Verification items for the finished model (mm, model axes). Give positions to 0.01 mm unless a question says otherwise; leave off trailing zeros. Order: outer loops, then holes, each group sorted by start corner. A loop starts at its lowest first (then second) coordinate and runs counter-clockwise, first axis right, second up. Notation, with made-up numbers: (75.25, 2.25) - (117.25, 2.25) arc R25 ccw to (117.25, 21.25) - close; hole circle Ø4 at (-5, 69.5). An arc over 180 degrees is marked (long way). Answer as a JSON object with one key per item and string values. Group by question number.
(1) Thickness scan on line 1 (Z direction, x = 28.5, y = 27); line 2 (Z direction, x = 5.5, y = -28.5); line 3 (X direction, y = 1, z = -116). Record the ranges inside material, lowest first.
(2) Section check A-A (z = 374.5). Record the boundary of the cut face in (x, y), then the cut area to 3 significant figures.
(3) Depth check by flat-ended pin: pin 1 Ø8 at (x, z) = (9.5, 32) entering from -Y; pin 2 Ø3 at (x, y) = (-28, -30.5) entering from -Z; pin 3 Ø5 at (y, z) = (-10.5, 190) entering from -X. Enter the tip coordinate at first touch or a pass-through.
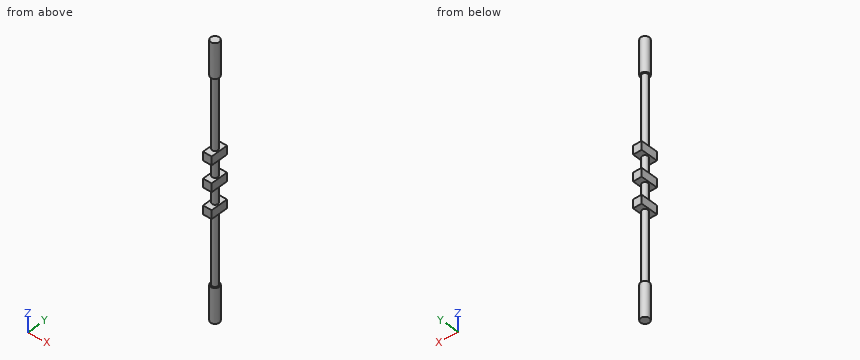
```python
from build123d import *

# Parameters (mm, degrees)
SKETCH1_R           = 25.4
BOSS_EXTRUDE1_DEPTH = 1778
SKETCH2_R           = 38.1
BOSS_EXTRUDE2_DEPTH = 304.8
BOSS_EXTRUDE3_START = 304.8
SKETCH3_R           = 38.1
BOSS_EXTRUDE3_DEPTH = 304.8
SKETCH4_W           = 76.2
SKETCH4_H           = 76.2
BOSS_EXTRUDE4_DEPTH = 76.2


with BuildPart() as part:
    # Sketch1 → Boss-Extrude1 (new body)
    with BuildSketch(Plane.XY):
        Circle(SKETCH1_R)
    extrude(amount=BOSS_EXTRUDE1_DEPTH)

    # Sketch2 → Boss-Extrude2 (add)
    with BuildSketch(Plane.XY.offset(1778)):
        with Locations(Location((0, 0, 0), (0, 0, 180))):
            Circle(SKETCH2_R)
    extrude(amount=BOSS_EXTRUDE2_DEPTH)

    # Sketch3 → Boss-Extrude3 (add)
    with BuildSketch(Plane(origin=(0, 0, 0), x_dir=(-1, 0, 0), z_dir=(0, 0, -1)).offset(BOSS_EXTRUDE3_START)):
        Circle(SKETCH3_R)
    extrude(amount=-BOSS_EXTRUDE3_DEPTH)

    # Sketch4 → Boss-Extrude4 (add, symmetric)
    with BuildSketch(Plane(origin=(0, 0, 0), x_dir=(1, 0, 0), z_dir=(0, 1, 0))):
        with Locations((0, -889)):
            Rectangle(SKETCH4_W, SKETCH4_H)
        with Locations((0, -1117.6)):
            Rectangle(SKETCH4_W, SKETCH4_H)
        with Locations((0, -660.4)):
            Rectangle(SKETCH4_W, SKETCH4_H)
    extrude(amount=BOSS_EXTRUDE4_DEPTH, both=True)


solid = part.part
```
Solutions:
{
 "1": {"line 1": "z = 622.3 to 698.5, 850.9 to 927.1, 1079.5 to 1155.7", "line 2": "z = -304.8 to 0, 622.3 to 698.5, 850.9 to 927.1, 1079.5 to 1155.7, 1778 to 2082.8", "line 3": "x = -38.09 to 38.09"},
 "2": {"outline": "circle Ø50.8 at (0, 0)", "area": "2,030 mm2"},
 "3": {"pin 1": "stops at y = -24.8", "pin 2": "stops at z = 622.3", "pin 3": "stops at x = -24.11"}
}
